Part model, mm, in its own coordinate system. A direction names the side the tool comes from. Coordinates: 2 decimals unless noted, no trailing zeros. Order: outer loops, then holes, each group sorted by start corner. A loop starts at its lowest first (then second) coordinate and runs counter-clockwise, first axis right, second up.
1) Wall check: L1, parallel to Y at x = 6.25, z = 0; L2, parallel to Y at x = -4.25, z = 0; L3, parallel to Z at x = 5.75, y = -14. Give the ranges that are in metal, low to high.
2) Cut at D-D (z = -14). List the corners of the cut face in (x, y), and give its area (3 significant figures).
3) Tool access for faces 5 (the flat face through (-8, -2, 5)), 6 (the cylindrical face through (4.93, -1.21, 14.815)), 7 (the cylindrical face through (4.93, 3.422, -14.514)), 8 (the cylindrical face through (4.93, -14.815, -1.21)), 9 (the cylindrical face through (4.93, -1.23, -14.86)): list every direction of +Z, -Z, +X, -X, +Y, -Y with a clear straight run to the whole face (end or side of a thin tool).
4) Pin check, flat tips, straight feed: pin 1 Ø4 at (y, z) = (-1, -11) entering from -X; pin 2 Ø1.2 at (x, z) = (-8, -6) entering from +Y; pin 3 Ø3 at (x, z) = (-6.5, 5) entering from -Y; pin 4 Ø1 at (y, z) = (-11, 6.5) entering from -X. Stop position of each tip, or through.
5) Cut at B-B (z = 0). List the corners of the cut face in (x, y), and give its area (3 significant figures).
6) Cut at A-A (y = 0). List the corners of the cut face in (x, z) (3 decimals).
7) Cut at C-C (x = -8). List the corners of the cut face in (y, z) (3 decimals), and give its area (3 significant figures).
8) Mould opens along Z. For faces 1 (the cylindrical face through (4.93, -9.687, 11.274)), 2 (the flat face through (-10, 4.3, 0.1)), 3 (the cylindrical face through (4.93, 7.73, 12.7)), 4 (the cylindrical face through (5, -6, -14)) say: +Z half, -Z half, draft (parallel to the pull), parting line (faces both ways), or undercut.
```python
from build123d import *

# Parameters (mm, degrees)
BASPROSKE_W        = 10
BASPROSKE_H        = 16.5
TOOTHCUT_DEPTH     = 26.38700455
TEETHCUTS_COUNT    = 20
TEETHCUTS_ANGLE    = 342
HUBNEAONESKE_R     = 10
HUBNEARONE_DEPTH   = 10.0000508
BORSKE_R           = 4
BORE_DEPTH         = 20.0000508
CUT_EXTRUDE1_DEPTH = 5


with BuildPart() as part:
    # BasProSke → Base-Revolve (revolve)
    with BuildSketch(Plane(origin=(0, 0, 0), x_dir=(1, 0, 0), z_dir=(0, 1, 0)), mode=Mode.PRIVATE) as base_revolve_sk:
        with Locations((5, 8.25)):
            Rectangle(BASPROSKE_W, BASPROSKE_H)
    revolve(base_revolve_sk.sketch.rotate(Axis((-10, 0, 0), (1, 0, 0)), 180), axis=Axis((-10, 0, 0), (1, 0, 0)))

    # TooCutSke → ToothCut (cut, through all)
    with BuildSketch(Plane(origin=(0, 0, 0), x_dir=(0, 0, -1), z_dir=(1, 0, 0))):
        with BuildLine():
            ThreePointArc((0.74381438, 13.102904875), (0, 13.124), (-0.74381438, 13.102904875))
            ThreePointArc((-0.74381438, 13.102904875), (-1.226473103, 14.852072512), (-2.209965745, 16.376962373))
            ThreePointArc((-2.209965745, 16.376962373), (0, 16.5254), (2.209965745, 16.376962373))
            ThreePointArc((2.209965745, 16.376962373), (1.226473103, 14.852072512), (0.74381438, 13.102904875))
        make_face()
    toothcut = extrude(amount=TOOTHCUT_DEPTH, mode=Mode.SUBTRACT)

    # TeethCuts: ToothCut ×20 about axis
    teethcuts_axis = Axis((-10, 0, 0), (1, 0, 0))
    for i in range(1, TEETHCUTS_COUNT):
        add(toothcut.rotate(teethcuts_axis, i * TEETHCUTS_ANGLE / (TEETHCUTS_COUNT - 1)), mode=Mode.SUBTRACT)

    # HubNeaOneSke → HubNearOne (add)
    with BuildSketch(Plane.ZY):
        with Locations(Location((0, 0, 0), (0, 0, 180))):
            Circle(HUBNEAONESKE_R)
    extrude(amount=HUBNEARONE_DEPTH)

    # BorSke → Bore (cut, symmetric)
    with BuildSketch(Plane(origin=(0, 0, 0), x_dir=(0, 0, -1), z_dir=(1, 0, 0))):
        with Locations(Location((0, 0, 0), (0, 0, 180))):
            Circle(BORSKE_R)
    extrude(amount=BORE_DEPTH, both=True, mode=Mode.SUBTRACT)

    # Sketch2 → Cut-Extrude1 (cut)
    with BuildSketch(Plane.ZY.offset(10.0000508)):
        with BuildLine():
            Line((3.12475599, -2), (7.445, -2))
            ThreePointArc((7.445, -2), (9.445, 0), (7.445, 2))
            Line((7.445, 2), (3.12475599, 2))
            ThreePointArc((3.12475599, 2), (0, 3.71), (-3.12475599, 2))
            Line((-3.12475599, 2), (-7.445, 2))
            ThreePointArc((-7.445, 2), (-9.445, 0), (-7.445, -2))
            Line((-7.445, -2), (-3.12475599, -2))
            ThreePointArc((-3.12475599, -2), (0, -3.71), (3.12475599, -2))
        make_face()
    extrude(amount=-CUT_EXTRUDE1_DEPTH, mode=Mode.SUBTRACT)


solid = part.part
```
Geometry check:
1. L1: y = -13.12 to -4, 4 to 13.12
1. L2: y = -10 to -4, 4 to 10
1. L3: z = -7.87 to -6, -3.46 to -0.92, 0.92 to 3.46, 6 to 7.87
2. outline: (0, -7.87) - (10, -7.87) - (10, -6) - (0, -6) - close; (0, -3.46) - (10, -3.46) - (10, -0.92) - (0, -0.92) - close; (0, 0.92) - (10, 0.92) - (10, 3.46) - (0, 3.46) - close; (0, 6) - (10, 6) - (10, 7.87) - (0, 7.87) - close
2. area: 88.1 mm2
3. face 5: -X
3. face 6: +Z, +X, -X
3. face 7: +X, -X
3. face 8: +X, -X, -Y
3. face 9: -Z, +X, -X
4. pin 1: stops at x = -10
4. pin 2: stops at y = 8.42
4. pin 3: stops at y = -9.37
4. pin 4: stops at x = 0
5. outline: (-10, -10) - (0, -10) - (0, -13.12) - (10, -13.12) - (10, -4) - (-10, -4) - close; (-10, 4) - (10, 4) - (10, 13.12) - (0, 13.12) - (0, 10) - (-10, 10) - close
5. area: 302 mm2
6. outline: (-10, -10) - (0, -10) - (0, -13.124) - (10, -13.124) - (10, -4) - (-5, -4) - (-5, -9.445) - (-10, -9.445) - close; (-10, 9.445) - (-5, 9.445) - (-5, 4) - (10, 4) - (10, 13.124) - (0, 13.124) - (0, 10) - (-10, 10) - close
7. outline: circle Ø20 at (0, 0); hole (-2, -7.445) arc R2 ccw to (2, -7.445) - (2, -3.464) arc R4 ccw to (2, 3.464) - (2, 7.445) arc R2 ccw to (-2, 7.445) - (-2, 3.464) arc R4 ccw to (-2, -3.464) - close
7. area: 222 mm2
8. face 1: +Z half
8. face 2: draft
8. face 3: undercut
8. face 4: -Z half
